Geometry: final body of the model. Coordinates: model frame, mm. Face numbers are marked on the shaded views. Give positions to 0.01 mm unless a question says otherwise; leave off trailing zeros. Write each loop counter-clockwise with the first axis right and the second up, starting at its lowest first coordinate (ties: lowest second). Pieces come first, ordered by that corner, then holes. Notation, with made-up numbers: M 10.25,-23 L 32.25,-23 A14 cw 32.25,1 Z; hole C -10.5,-21.5 d9. An arc over 180 degrees is marked long. Use a Markdown table: item, result. Add a question column.
(1) Pin query (flat end, axial travel): pin 1 Ø1 at (x, z) = (-29.5, -19.5) entering from +Y. Return the tip coordinate at first contact, or that it passes through.
(2) Cut plane D-D (x = 0). Output: boundary loops of the cut face in (y, z), plus the area to 3 significant figures.
(3) Draft query along X for the marked faces 1 and 2. Return one class per face: released by +X, released by -X, zero draft, split by the parting line, or undercut.
(4) Cut plane C-C (z = 14). Output: boundary loops of the cut face in (x, y).
(5) Cut plane B-B (y = 4.3). Output: boundary loops of the cut face in (x, z), plus the area to 3 significant figures.
(6) Cut plane A-A (x = -47.5). Output: boundary loops of the cut face in (y, z).
(7) Material intervals for L1, parallel to X at y = 1.35, z = -24; L2, parallel to Y at x = 18, z = -18.5, sorted ascending.
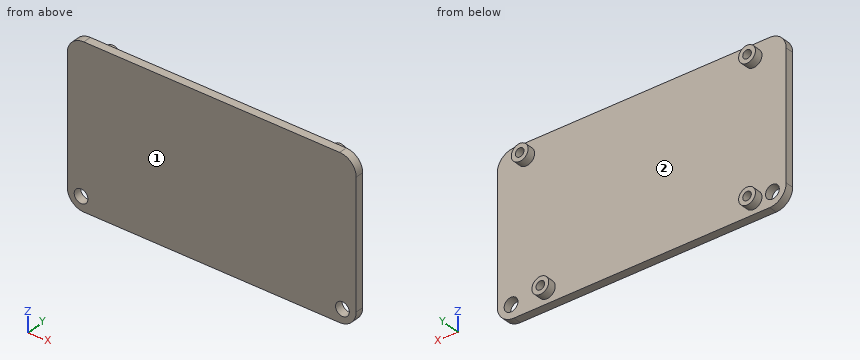
Autodesk Inventor part; units mm, degrees
ref_plane "YZ Plane" through (0, 0, 0) normal (1, 0, 0) x (0, 1, 0)
ref_plane "XZ Plane" through (0, 0, 0) normal (0, 1, 0) x (-1, 0, 0)
ref_plane "XY Plane" through (0, 0, 0) normal (0, 0, 1) x (1, 0, 0)
sketch "Sketch1" plane through (0, 0, 0) normal (0, 1, 0) x (-1, 0, 0)
  line L0 (52.5, 29) -> (-52.5, 29)
  line L1 (-52.5, 29) -> (-52.5, -29)
  line L2 (-52.5, -29) -> (52.5, -29)
  line L3 (52.5, -29) -> (52.5, 29)
  line L4 (52.5, 29) -> (-52.5, -29) construction
  line L5 (-52.5, 29) -> (52.5, -29) construction
  point P0 (0, 0)
  dimension "d0" = 105
  dimension "d1" = 58
extrude "Extrusion1" add sketch "Sketch1" along normal blind 3
sketch "Sketch2" plane through (0, 3, 0) normal (0, 1, 0) x (1, 0, 0)
  circle A0 centre (41.9878, -24.0965) radius 1.562
  circle A1 centre (41.9878, -24.0965) radius 3.062
  circle A2 centre (-40.6382, -24.0965) radius 1.562
  circle A3 centre (-40.6382, -24.0965) radius 3.062
  circle A4 centre (-40.6382, 24.2395) radius 1.562
  circle A5 centre (-40.6382, 24.2395) radius 3.062
  circle A6 centre (34.4948, 24.2395) radius 1.562
  circle A7 centre (34.4948, 24.2395) radius 3.062
  point P0 (0, 0)
  dimension "d4" = 3.124
  dimension "d5" = 1.5
  dimension "d6" = 3.124
  dimension "d7" = 1.5
  dimension "d8" = 82.626
  dimension "d9" = 3.124
  dimension "d10" = 1.5
  dimension "d11" = 48.336
  dimension "d12" = 3.124
  dimension "d13" = 1.5
  dimension "d14" = 75.133
  dimension "d15" = 0
  dimension "d16" = 0
extrude "Extrusion2" add sketch "Sketch2" along normal blind 3
sketch "Sketch3" plane through (0, 3, 0) normal (0, 1, 0) x (1, 0, 0)
  circle A0 centre (47.5, 24) radius 2.5
  line L0 (52.5, 29) -> (-52.5, 29)
  line L1 (52.5, -29) -> (52.5, 29)
  circle A1 centre (-47.5, 24) radius 2.5
  line L2 (-52.5, 29) -> (-52.5, -29)
  point P0 (0, 0)
  dimension "d19" = 5
  dimension "d20" = 5
  dimension "d21" = 5
  dimension "d22" = 5
  dimension "d23" = 5
  dimension "d24" = 5
extrude "Extrusion3" cut sketch "Sketch3" against normal through all
fillet "Fillet1" radius 6 4 edges at (52.5, 1.5, 29) (52.5, 1.5, -29) (-52.5, 1.5, 29) (-52.5, 1.5, -29)
properties part number "placa_arduino"
Answer list:
| question | item | result |
|---|---|---|
| 1 | pin 1 | y = 3 |
| 2 | outline | M 0,-29 L 3,-29 L 3,29 L 0,29 Z |
| 2 | area | 174 mm² |
| 3 | face 1 | zero draft |
| 3 | face 2 | undercut |
| 4 | outline | M -52.5,0 L 52.5,0 L 52.5,3 L -52.5,3 Z |
| 5 | outline | C -40.64,-24.24 d6.12; C -40.64,24.1 d6.12; C 34.49,-24.24 d6.12; C 41.99,24.1 d6.12; hole C -40.64,-24.24 d3.12; hole C -40.64,24.1 d3.12; hole C 34.49,-24.24 d3.12; hole C 41.99,24.1 d3.12 |
| 5 | area | 87.2 mm² |
| 6 | outline | M 0,-28.92 L 3,-28.92 L 3,-26.5 L 0,-26.5 Z; M 0,-21.5 L 3,-21.5 L 3,28.92 L 0,28.92 Z |
| 7 | L1 | -52.42 to -50, -45 to 45, 50 to 52.42 |
| 7 | L2 | 0 to 3 |
